Geometry check sheet. Reference: drawing and pictorial views, mm from the part's lowest x, y, z. Round coordinates to 2 decimals unless told otherwise and drop trailing zeros. Order: outer loops, then holes, each group sorted by start corner. A loop starts at its lowest first (then second) coordinate and runs counter-clockwise, first axis right, second up.
Q1. Cross-section at D-D on x = 9. Record the cut outline in (y, z), then the cut area to 3 significant figures.
Q2. Cross-section at A-A on y = 10. Record the cut outline in (x, z).
Q3. Cross-section at C-C on z = 0.7. Record the cut outline in (x, y), then the cut area to 3 significant figures.
Q4. Cross-section at B-B on x = 35. Record the cut outline in (y, z).
Q5. Scan lines: probe 1 along X at (y, z) = (10, 0.45); probe 2 along Y at (x, z) = (35, 0.7); probe 3 along X at (y, z) = (8, 0.6). Record each from-to range of solid material in increasing order.
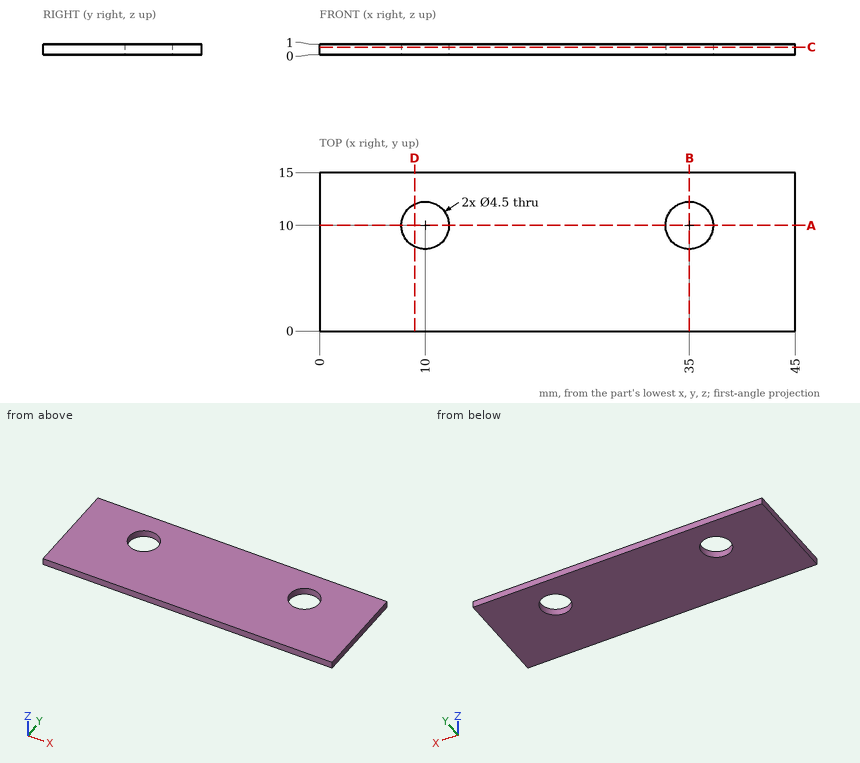
Results found:
1. outline: (0, 0) - (7.98, 0) - (7.98, 1) - (0, 1) - close; (12.02, 0) - (15, 0) - (15, 1) - (12.02, 1) - close
1. area: 11.0 mm2
2. outline: (0, 0) - (7.75, 0) - (7.75, 1) - (0, 1) - close; (12.25, 0) - (32.75, 0) - (32.75, 1) - (12.25, 1) - close; (37.25, 0) - (45, 0) - (45, 1) - (37.25, 1) - close
3. outline: (0, 0) - (45, 0) - (45, 15) - (0, 15) - close; hole circle Ø4.5 at (10, 10); hole circle Ø4.5 at (35, 10)
3. area: 643 mm2
4. outline: (0, 0) - (7.75, 0) - (7.75, 1) - (0, 1) - close; (12.25, 0) - (15, 0) - (15, 1) - (12.25, 1) - close
5. probe 1: x = 0 to 7.75, 12.25 to 32.75, 37.25 to 45
5. probe 2: y = 0 to 7.75, 12.25 to 15
5. probe 3: x = 0 to 8.97, 11.03 to 33.97, 36.03 to 45
